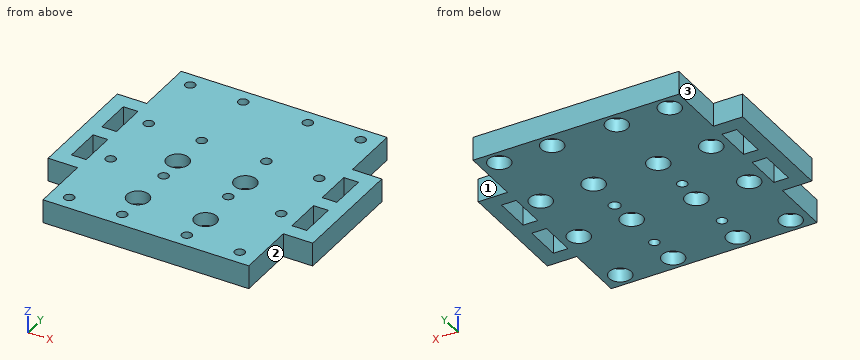
```python
from build123d import *

# Parameters (mm, degrees)
SKETCH_1_W          = 70
SKETCH_1_H          = 80
SKETCH_1_R          = 1.7
EXTRUDE_1_DEPTH     = 8
SKETCH_2_R          = 3.75
CUT_EXTRUDE_1_DEPTH = 4.5
EXTRUDE_2_DEPTH     = 8
SKETCH_4_R          = 1.7
CUT_EXTRUDE_2_DEPTH = 20
SKETCH_6_R          = 3.75
CUT_EXTRUDE_4_DEPTH = 4.5
SKETCH_7_R          = 1.938201366
SKETCH_7_R_2        = 1.7
CUT_EXTRUDE_5_DEPTH = 10
SKETCH_8_R          = 3.75
CUT_EXTRUDE_6_DEPTH = 4.5


with BuildPart() as part:
    # 草图1 → 凸台-拉伸1 (new body)
    with BuildSketch(Plane.XY):
        with Locations((2.682119205, -17.951221502)):
            Rectangle(SKETCH_1_W, SKETCH_1_H)
        with Locations((-26.317880795, 17.048778498)):
            Circle(SKETCH_1_R, mode=Mode.SUBTRACT)
        with Locations((-8.317880795, 17.048778498)):
            Circle(SKETCH_1_R, mode=Mode.SUBTRACT)
        with Locations((-26.317880795, -6.951221502)):
            Circle(SKETCH_1_R, mode=Mode.SUBTRACT)
        with Locations((-8.317880795, -6.951221502)):
            Circle(SKETCH_1_R, mode=Mode.SUBTRACT)
        with Locations(Location((31.682119205, -6.951221502, 0), (0, 0, 180))):
            Circle(SKETCH_1_R, mode=Mode.SUBTRACT)
        with Locations(Location((13.682119205, -6.951221502, 0), (0, 0, 180))):
            Circle(SKETCH_1_R, mode=Mode.SUBTRACT)
        with Locations(Location((13.682119205, 17.048778498, 0), (0, 0, 180))):
            Circle(SKETCH_1_R, mode=Mode.SUBTRACT)
        with Locations(Location((31.682119205, 17.048778498, 0), (0, 0, 180))):
            Circle(SKETCH_1_R, mode=Mode.SUBTRACT)
        with Locations((13.682119205, -28.951221502)):
            Circle(SKETCH_1_R, mode=Mode.SUBTRACT)
        with Locations((31.682119205, -28.951221502)):
            Circle(SKETCH_1_R, mode=Mode.SUBTRACT)
        with Locations((31.682119205, -52.951221502)):
            Circle(SKETCH_1_R, mode=Mode.SUBTRACT)
        with Locations((13.682119205, -52.951221502)):
            Circle(SKETCH_1_R, mode=Mode.SUBTRACT)
        with Locations(Location((-26.317880795, -28.951221502, 0), (0, 0, 180))):
            Circle(SKETCH_1_R, mode=Mode.SUBTRACT)
        with Locations(Location((-8.317880795, -28.951221502, 0), (0, 0, 180))):
            Circle(SKETCH_1_R, mode=Mode.SUBTRACT)
        with Locations(Location((-8.317880795, -52.951221502, 0), (0, 0, 180))):
            Circle(SKETCH_1_R, mode=Mode.SUBTRACT)
        with Locations(Location((-26.317880795, -52.951221502, 0), (0, 0, 180))):
            Circle(SKETCH_1_R, mode=Mode.SUBTRACT)
    extrude(amount=EXTRUDE_1_DEPTH)

    # 草图2 → 切除-拉伸1 (cut)
    with BuildSketch(Plane(origin=(0, 0, 0), x_dir=(-1, 0, 0), z_dir=(0, 0, -1))):
        with Locations((-31.682119205, 17.048778498)):
            Circle(SKETCH_2_R)
        with Locations((-13.682119205, 17.048778498)):
            Circle(SKETCH_2_R)
        with Locations((8.317880795, 17.048778498)):
            Circle(SKETCH_2_R)
        with Locations((26.317880795, 17.048778498)):
            Circle(SKETCH_2_R)
        with Locations((-31.682119205, -6.951221502)):
            Circle(SKETCH_2_R)
        with Locations((-13.682119205, -6.951221502)):
            Circle(SKETCH_2_R)
        with Locations((8.317880795, -6.951221502)):
            Circle(SKETCH_2_R)
        with Locations((26.317880795, -6.951221502)):
            Circle(SKETCH_2_R)
        with Locations(Location((-31.682119205, -28.951221502, 0), (0, 0, 180))):
            Circle(SKETCH_2_R)
        with Locations(Location((-13.682119205, -28.951221502, 0), (0, 0, 180))):
            Circle(SKETCH_2_R)
        with Locations(Location((8.317880795, -28.951221502, 0), (0, 0, 180))):
            Circle(SKETCH_2_R)
        with Locations(Location((26.317880795, -28.951221502, 0), (0, 0, 180))):
            Circle(SKETCH_2_R)
        with Locations(Location((26.317880795, -52.951221502, 0), (0, 0, 180))):
            Circle(SKETCH_2_R)
        with Locations(Location((8.317880795, -52.951221502, 0), (0, 0, 180))):
            Circle(SKETCH_2_R)
        with Locations(Location((-13.682119205, -52.951221502, 0), (0, 0, 180))):
            Circle(SKETCH_2_R)
        with Locations(Location((-31.682119205, -52.951221502, 0), (0, 0, 180))):
            Circle(SKETCH_2_R)
    extrude(amount=-CUT_EXTRUDE_1_DEPTH, mode=Mode.SUBTRACT)

    # 草图3 → 凸台-拉伸2 (add)
    with BuildSketch(Plane.XY.offset(8)):
        Polygon((47.682119205, 2.048778498), (37.682119205, 2.048778498), (37.682119205, -2.951221502), (42.682119205, -2.951221502), (42.682119205, -15.451221502), (37.682119205, -15.451221502), (37.682119205, -20.451221502), (42.682119205, -20.451221502), (42.682119205, -32.951221502), (37.682119205, -32.951221502), (37.682119205, -37.951221502), (47.682119205, -37.951221502), align=None)
        Polygon((-32.317880795, -37.951221502), (-32.317880795, -32.951221502), (-37.317880795, -32.951221502), (-37.317880795, -20.451221502), (-32.317880795, -20.451221502), (-32.317880795, -15.451221502), (-37.317880795, -15.451221502), (-37.317880795, -2.951221502), (-32.317880795, -2.951221502), (-32.317880795, 2.048778498), (-42.317880795, 2.048778498), (-42.317880795, -37.951221502), align=None)
    extrude(amount=-EXTRUDE_2_DEPTH)

    # 草图4 → 切除-拉伸2 (cut)
    with BuildSketch(Plane.XY.offset(8)):
        with Locations((-8.817880795, -42.951221502)):
            Circle(SKETCH_4_R)
        with Locations((14.182119205, -42.951221502)):
            Circle(SKETCH_4_R)
    extrude(amount=-CUT_EXTRUDE_2_DEPTH, mode=Mode.SUBTRACT)

    # 草图6 → 切除-拉伸4 (cut)
    with BuildSketch(Plane.XY.offset(8)):
        with Locations((-8.817880795, -42.951221502)):
            Circle(SKETCH_6_R)
        with Locations((14.182119205, -42.951221502)):
            Circle(SKETCH_6_R)
    extrude(amount=-CUT_EXTRUDE_4_DEPTH, mode=Mode.SUBTRACT)

    # 草图7 → 切除-拉伸5 (cut)
    with BuildSketch(Plane(origin=(0, 0, 0), x_dir=(-1, 0, 0), z_dir=(0, 0, -1))):
        with Locations((-14.182119205, -19.951221502)):
            Circle(SKETCH_7_R)
        with Locations((8.817880795, -19.951221502)):
            Circle(SKETCH_7_R_2)
    extrude(amount=-CUT_EXTRUDE_5_DEPTH, mode=Mode.SUBTRACT)

    # 草图8 → 切除-拉伸6 (cut)
    with BuildSketch(Plane.XY.offset(8)):
        with Locations((-8.817880795, -19.951221502)):
            Circle(SKETCH_8_R)
        with Locations((14.182119205, -19.951221502)):
            Circle(SKETCH_8_R)
    extrude(amount=-CUT_EXTRUDE_6_DEPTH, mode=Mode.SUBTRACT)


solid = part.part
```
Here's how the part is built. I have some questions about the finished solid (model axes, mm). Face numbers are marked on the shaded views. A direction names the side the tool comes from. Coordinates: 2 decimals unless noted, no trailing zeros. Order: outer loops, then holes, each group sorted by start corner. A loop starts at its lowest first (then second) coordinate and runs counter-clockwise, first axis right, second up. Notation, with made-up numbers: M -14.5,59.5 L 38.5,59.5 A18 ccw 38.5,68.5 Z; hole C -16,13.5 d7. An arc over 180 degrees is marked long. Answer as a JSON object with one key per item and string values. Group by question number.
(1) Suppose I cut it at A-A, the plane x = 39.5. Please give me the cut outline in (y, z), then the cut area to 3 significant figures.
(2) Which directions (+Z, -Z, +X, -X, +Y, -Y) give clear straight access to the entire face, cutting with the end or side of a thin tool? Please do the marked faces 1, 2 and 3.
(3) For pin 1 (4 mm diameter, centred on x = 13.68, y = -6.95, fed in from -Z); pin 2 (2 mm diameter, centred on x = -8.32, y = -6.95, fed in from +Z); pin 3 (4.5 mm diameter, centred on x = 14.18, y = -42.95, fed in from +Z); pin 4 (4 mm diameter, centred on y = -43, z = 1.5, fed in from +X), each with a flat end and sliding along its axis, tell me the tip position at first contact or that it passes through.
(4) I need wall thicknesses on probe 1 along Y at (x, z) = (-35, 5); probe 2 along X at (y, z) = (-27, 7.5); probe 3 along X at (y, z) = (-20.5, 6.75). Which ranges of each line are inside material? Lowest first, please.
(5) Suppose I cut it at B-B, the plane y = 4. Please give me the cut outline in (x, z), then the cut area to 3 significant figures.
(6) Suppose I cut it at C-C, the plane z = 5.75. State how many separate pieces and enclosed holes the cut face has, then the cut area to 3 significant figures.
Values found:
{
 "1": {"outline": "M -37.95,0 L -32.95,0 L -32.95,8 L -37.95,8 Z; M -20.45,0 L -15.45,0 L -15.45,8 L -20.45,8 Z; M -2.95,0 L 2.05,0 L 2.05,8 L -2.95,8 Z", "area": "120 mm^2"},
 "2": {"face 1": "+Z, -Z, +X, +Y", "face 2": "+Z, -Z, +X, -Y", "face 3": "+Z, -Z, -X, +Y"},
 "3": {"pin 1": "stops at z = 4.5", "pin 2": "passes through", "pin 3": "stops at z = 3.5", "pin 4": "stops at x = 37.68"},
 "4": {"probe 1": "y = -37.95 to -32.95, -20.45 to -15.45, -2.95 to 2.05", "probe 2": "x = -42.32 to -37.32, -32.32 to 37.68, 42.68 to 47.68", "probe 3": "x = -42.32 to -37.32, -32.32 to -12.53, -5.11 to 10.47, 17.89 to 37.68, 42.68 to 47.68"},
 "5": {"outline": "M -32.32,0 L 37.68,0 L 37.68,8 L -32.32,8 Z", "area": "560 mm^2"},
 "6": {"separate pieces": "1", "enclosed holes": "24", "area": "5,830 mm^2"}
}
